from build123d import *

# Parameters (mm, degrees)
PAD_DEPTH       = 67
SKETCH001_R     = 1.8
POCKET_DEPTH    = 5
SKETCH002_W     = 36.32
SKETCH002_H     = 47
POCKET001_DEPTH = 5
SKETCH003_W     = 36.32
SKETCH003_H     = 47
POCKET002_DEPTH = 5
FILLET_R        = 4
PAD001_DEPTH    = 4
PAD002_DEPTH    = 4
SKETCH006_W     = 8
SKETCH006_H     = 33
POCKET003_DEPTH = 100


with BuildPart() as part:
    # Sketch → Pad (new body)
    with BuildSketch(Plane.XY):
        Polygon((20, 22), (24, 22), (24, 0), (24, -3), (0, -43), (-24, -3), (-24, 0), (-24, 22), (-20, 22), (-8, 22), (-8, 18), (-20, 18), (-20, 0), (0, -35), (20, 0), (20, 18), (8, 18), (8, 22), align=None)
    extrude(amount=PAD_DEPTH)

    # Sketch001 (on Face10 of Pad) → Pocket (cut)
    with BuildSketch(Plane(origin=(0, 22, 0), x_dir=(-1, 0, 0), z_dir=(0, 1, 0))):
        with Locations((15, 56.5)):
            Circle(SKETCH001_R)
        with Locations((15, 10.5)):
            Circle(SKETCH001_R)
        with Locations((-15, 56.5)):
            Circle(SKETCH001_R)
        with Locations((-15, 10.5)):
            Circle(SKETCH001_R)
    extrude(amount=-POCKET_DEPTH, mode=Mode.SUBTRACT)

    # Sketch002 (on Face11 of Pocket) → Pocket001 (cut)
    with BuildSketch(Plane(origin=(-18.9705882353, -11.3823529412, 0), x_dir=(0.5144957554, -0.8574929257, 0), z_dir=(-0.8574929257, -0.5144957554, 0))):
        with Locations((7.84, 33.5)):
            Rectangle(SKETCH002_W, SKETCH002_H)
    extrude(amount=-POCKET001_DEPTH, mode=Mode.SUBTRACT)

    # Sketch003 (on Face10 of Pocket001) → Pocket002 (cut)
    with BuildSketch(Plane(origin=(18.9705882353, -11.3823529412, 0), x_dir=(0.5144957554, 0.8574929257, 0), z_dir=(0.8574929257, -0.5144957554, 0))):
        with Locations((-7.84, 33.5)):
            Rectangle(SKETCH003_W, SKETCH003_H)
    extrude(amount=-POCKET002_DEPTH, mode=Mode.SUBTRACT)

    # Fillet
    fillet_edges = [part.edges().sort_by_distance(p)[0] for p in [
        (0, -43, 33.5),
    ]]
    fillet(fillet_edges, radius=FILLET_R)

    # Sketch004 (on Face19 of Pad) → Pad001 (join)
    with BuildSketch(Plane(origin=(0, 0, 0), x_dir=(1, 0, 0), z_dir=(0, 0, -1))):
        Polygon((24, 3), (24, -6), (-24, -6), (-24, 3), (-11.4, 24), (11.4, 24), align=None)
    extrude(amount=PAD001_DEPTH)

    # Sketch005 → Pad002 (join)
    with BuildSketch(Plane.XY.offset(67)):
        Polygon((13.8, -20), (-13.8, -20), (-11.4, -24), (11.4, -24), align=None)
    extrude(amount=PAD002_DEPTH)

    # Sketch006 (on Face17 of Pad002) → Pocket003 (cut)
    with BuildSketch(Plane(origin=(-24, 0, 0), x_dir=(0, -1, 0), z_dir=(-1, 0, 0))):
        with Locations((-18, 33.5)):
            Rectangle(SKETCH006_W, SKETCH006_H)
    extrude(amount=-POCKET003_DEPTH, mode=Mode.SUBTRACT)


solid = part.part
Source: CAD feature listing. Evaluate the final solid. Frame: model axes, mm. A direction names the side the tool comes from. Give positions to 0.01 mm unless a question says otherwise; leave off trailing zeros. Write each loop counter-clockwise with the first axis right and the second up, starting at its lowest first coordinate (ties: lowest second). Pieces come first, ordered by that corner, then holes. Notation, with made-up numbers: M 56.5,13.5 L 65.5,13.5 A16 cw 65.5,34.5 Z; hole C 76,20 d4. An arc over 180 degrees is marked long. Return JSON: item names as keys, results as strings. Group by question number.
1) Set-up query: faces 1 (the face through (-21, 4, 67)), 2 (the face through (22, 14, 33)), 3 (the face through (0, -24, -2)), 4 (the face through (-8, 20, 8)). Return all of +Z, -Z, +X, -X, +Y, -Y with unobstructed straight access to the full face (end or side cutting, diameter ignored); none if empty.
2) Cut plane B-B, the plane x = -15. Output: boundary loops of the cut face in (y, z), then the cut area to 3 significant figures.
3) Draft query along Y for faces 5 (the face through (21, 18, 0)), 6 (the face through (0, -20, 69)), 7 (the face through (-1.899, -31.678, 35.825)). Return one class per face: released by +Y, released by -Y, zero draft, split by the parting line, or undercut.
4) Ray query, L1, parallel to Z at x = -15, y = 21; L2, parallel to Z at x = 21, y = 15; L3, parallel to X at y = 12, z = 64. Return the intervals inside material, ascending.
5) Cut plane C-C, the plane y = 15. Output: boundary loops of the cut face in (x, z).
6) Cut plane D-D, the plane x = 18. Output: boundary loops of the cut face in (y, z).
7) First-contact query: pin 1 Ø8 at (x, y) = (-17, 7.5) entering from +Z; pin 2 Ø2.5 at (x, y) = (15, 16.5) entering from +Z; pin 3 Ø3.5 at (x, z) = (11.5, 9) entering from -Y; pin 4 Ø1 at (x, z) = (3, 31.5) entering from +Y. Flat tips, straight axial feed; report the tip coordinate or a pass-through.
8) Cut plane A-A, the plane z = 44.5. Output: boundary loops of the cut face in (x, y), then the cut area to 3 significant figures.
Data:
{
 "1": {"face 1": "+Z, +X, -X, +Y", "face 2": "+X, -X, +Y", "face 3": "-Z, +X, -X, -Y", "face 4": "+Z, -Z, +Y"},
 "2": {"outline": "M -18,-4 L 6,-4 L 6,0 L -8.75,0 L -8.75,10 L -18,10 Z; M -18,57 L -8.75,57 L -8.75,67 L -18,67 Z; M 18,0 L 22,0 L 22,8.7 L 18,8.7 Z; M 18,12.3 L 22,12.3 L 22,17 L 18,17 Z; M 18,50 L 22,50 L 22,54.7 L 18,54.7 Z; M 18,58.3 L 22,58.3 L 22,67 L 18,67 Z", "area": "388 mm²"},
 "3": {"face 5": "zero draft", "face 6": "released by +Y", "face 7": "undercut"},
 "4": {"L1": "z = 0 to 8.7, 12.3 to 17, 50 to 54.7, 58.3 to 67", "L2": "z = 0 to 17, 50 to 67", "L3": "x = -24 to -20, 20 to 24"},
 "5": {"outline": "M -24,0 L -20,0 L -20,17 L -24,17 Z; M -24,50 L -20,50 L -20,67 L -24,67 Z; M 20,0 L 24,0 L 24,17 L 20,17 Z; M 20,50 L 24,50 L 24,67 L 20,67 Z"},
 "6": {"outline": "M -13,-4 L 6,-4 L 6,0 L -3.5,0 L -3.5,10 L -13,10 Z; M -13,57 L -3.5,57 L -3.5,67 L -13,67 Z; M 18,0 L 22,0 L 22,17 L 18,17 Z; M 18,50 L 22,50 L 22,67 L 18,67 Z"},
 "7": {"pin 1": "stops at z = 67", "pin 2": "passes through", "pin 3": "stops at y = -26.75", "pin 4": "stops at y = -31.82"},
 "8": {"outline": "M -24,-2.36 L -20,0.04 L -20,14 L -24,14 Z; M -5.59,-33.68 L -3.43,-37.28 A4 ccw 3.43,-37.28 L 5.59,-33.68 L 1.99,-31.52 L 0,-35 L -1.99,-31.52 Z; M 20,0.04 L 24,-2.36 L 24,14 L 20,14 Z", "area": "173 mm²"}
}
